```python
from build123d import *

# Parameters (mm, degrees)
SKETCH1_R                = 2.5
F_20_X_20_X_R1_5_1_DEPTH = 100


with BuildPart() as part:
    # Sketch1 → 铝型材 20 X 20 X R1.5(1) (new body)
    with BuildSketch(Plane.YX):
        with BuildLine():
            Line((-3.6, 10), (-3.6, 9.5))
            Line((-3.6, 9.5), (-3.1, 9.5))
            Line((-3.1, 9.5), (-3.1, 8.5))
            Line((-3.1, 8.5), (-5.5, 8.5))
            Line((-5.5, 8.5), (-5.5, 6.65))
            Line((-5.5, 6.65), (-2.75, 3.9))
            Line((-2.75, 3.9), (2.75, 3.9))
            Line((2.75, 3.9), (5.5, 6.65))
            Line((5.5, 6.65), (5.5, 8.5))
            Line((5.5, 8.5), (3.1, 8.5))
            Line((3.1, 8.5), (3.1, 9.5))
            Line((3.1, 9.5), (3.6, 9.5))
            Line((3.6, 9.5), (3.6, 10))
            Line((3.6, 10), (8.5, 10))
            ThreePointArc((8.5, 10), (9.560660172, 9.560660172), (10, 8.5))
            Line((10, 8.5), (10, 3.6))
            Line((10, 3.6), (9.5, 3.6))
            Line((9.5, 3.6), (9.5, 3.1))
            Line((9.5, 3.1), (8.5, 3.1))
            Line((8.5, 3.1), (8.5, 5.5))
            Line((8.5, 5.5), (6.65, 5.5))
            Line((6.65, 5.5), (3.9, 2.75))
            Line((3.9, 2.75), (3.9, -2.75))
            Line((3.9, -2.75), (6.65, -5.5))
            Line((6.65, -5.5), (8.5, -5.5))
            Line((8.5, -5.5), (8.5, -3.1))
            Line((8.5, -3.1), (9.5, -3.1))
            Line((9.5, -3.1), (9.5, -3.6))
            Line((9.5, -3.6), (10, -3.6))
            Line((10, -3.6), (10, -8.5))
            ThreePointArc((10, -8.5), (9.560660172, -9.560660172), (8.5, -10))
            Line((8.5, -10), (3.6, -10))
            Line((3.6, -10), (3.6, -9.5))
            Line((3.6, -9.5), (3.1, -9.5))
            Line((3.1, -9.5), (3.1, -8.5))
            Line((3.1, -8.5), (5.5, -8.5))
            Line((5.5, -8.5), (5.5, -6.65))
            Line((5.5, -6.65), (2.75, -3.9))
            Line((2.75, -3.9), (-2.75, -3.9))
            Line((-2.75, -3.9), (-5.5, -6.65))
            Line((-5.5, -6.65), (-5.5, -8.5))
            Line((-5.5, -8.5), (-3.1, -8.5))
            Line((-3.1, -8.5), (-3.1, -9.5))
            Line((-3.1, -9.5), (-3.6, -9.5))
            Line((-3.6, -9.5), (-3.6, -10))
            Line((-3.6, -10), (-8.5, -10))
            ThreePointArc((-8.5, -10), (-9.560660172, -9.560660172), (-10, -8.5))
            Line((-10, -8.5), (-10, -3.6))
            Line((-10, -3.6), (-9.5, -3.6))
            Line((-9.5, -3.6), (-9.5, -3.1))
            Line((-9.5, -3.1), (-8.5, -3.1))
            Line((-8.5, -3.1), (-8.5, -5.5))
            Line((-8.5, -5.5), (-6.65, -5.5))
            Line((-6.65, -5.5), (-3.9, -2.75))
            Line((-3.9, -2.75), (-3.9, 2.75))
            Line((-3.9, 2.75), (-6.65, 5.5))
            Line((-6.65, 5.5), (-8.5, 5.5))
            Line((-8.5, 5.5), (-8.5, 3.1))
            Line((-8.5, 3.1), (-9.5, 3.1))
            Line((-9.5, 3.1), (-9.5, 3.6))
            Line((-9.5, 3.6), (-10, 3.6))
            Line((-10, 3.6), (-10, 8.5))
            ThreePointArc((-10, 8.5), (-9.560660172, 9.560660172), (-8.5, 10))
            Line((-8.5, 10), (-3.6, 10))
        make_face()
        Circle(SKETCH1_R, mode=Mode.SUBTRACT)
    extrude(amount=F_20_X_20_X_R1_5_1_DEPTH)


solid = part.part
```
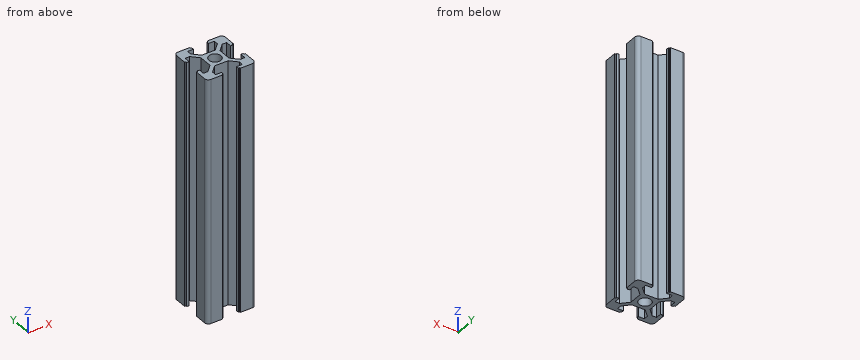
Work out the finished part from the listing and answer in its coordinate system (mm). Give positions to 0.01 mm unless a question says otherwise; leave off trailing zeros. Loops run counter-clockwise (first coordinate to the right, second up) from the corner with the lowest first, then second, coordinate; pieces in that order, holes last. Notation, with made-up numbers: (34, 42) - (77, 42) arc R9 ccw to (77, 56) - close; hole circle Ø5 at (44.25, 65). An arc over 180 degrees is marked (long way). Use CSV: the item, a comma, the result in double quotes. Start each with the question number.
(1) Each of these flat-tipped pins is pushed along its axis until it touches: pin 1 (0.8 mm diameter, centred on y = 9, z = -52.5, fed in from -X); pin 2 (0.8 mm diameter, centred on y = -9, z = -41.5, fed in from +X); pin 3 (6 mm diameter, centred on x = 0, z = -45.5, fed in from +Y). Where does it stop, or does it pass through?
(2) Find the intervals of material crossed by L1, parallel to X at y = 0, z = -61.5; L2, parallel to X at y = -8.25, z = -96; L3, parallel to X at y = 3.5, z = -32, in increasing order.
(3) Find section A-A, the plane y = 7.5. Determine the outline of the cut face in (x, z).
(4) Find section B-B, the plane x = 0. Determine the outline of the cut face in (y, z).
Results found:
1,pin 1,"x = -10"
1,pin 2,"x = 10"
1,pin 3,"y = 4.15"
2,L1,"-3.9 to -2.5, 2.5 to 3.9"
2,L2,"-10 to -5.5, 5.5 to 10"
2,L3,"-9.5 to -8.5, -4.65 to 4.65, 8.5 to 9.5"
3,outline,"(-10, -100) - (-5.5, -100) - (-5.5, 0) - (-10, 0) - close; (5.5, -100) - (10, -100) - (10, 0) - (5.5, 0) - close"
4,outline,"(-3.9, -100) - (-2.5, -100) - (-2.5, 0) - (-3.9, 0) - close; (2.5, -100) - (3.9, -100) - (3.9, 0) - (2.5, 0) - close"
